from build123d import *

# Parameters (mm, degrees)
SKETCH_1_W               = 11
SKETCH_1_H               = 6.169
CUT_EXTRUDE_2_REACH      = 19.004
PATTERN_CIRCULAR_3_COUNT = 20
EXTRUDE_START            = 2
SKETCH_7_R               = 11
SKETCH_7_R_2             = 3
EXTRUDE_1_DEPTH          = 2
EXTRUDE_START_2          = -11
SKETCH_7_2_R             = 11
SKETCH_7_2_R_2           = 3
EXTRUDE_2_DEPTH          = 2
CHAMFER_1_SIZE           = 0.5


with BuildPart() as part:
    # 草图1 → 旋转1 (revolve)
    with BuildSketch(Plane.XY, mode=Mode.PRIVATE) as revolve_1_sk:
        with Locations((5.5, 6.0845)):
            Rectangle(SKETCH_1_W, SKETCH_1_H)
    revolve(revolve_1_sk.sketch.rotate(Axis((0, 0, 0), (1, 0, 0)), 90), axis=Axis((0, 0, 0), (1, 0, 0)))

    # 草图6 → 切除-拉伸2 (cut, up to next)
    with BuildSketch(Plane(origin=(0, 0, 0), x_dir=(0, 0, -1), z_dir=(1, 0, 0)), mode=Mode.PRIVATE) as cut_extrude_2_sk1:
        with BuildLine():
            Line((0.924550348, 8.86184509), (0.903216998, 8.688098898))
            ThreePointArc((0.903216998, 8.688098898), (0, 7.889), (-0.903216998, 8.688098898))
            Line((-0.903216998, 8.688098898), (-0.924550348, 8.86184509))
            ThreePointArc((-0.924550348, 8.86184509), (-1.023665877, 9.035916247), (-1.217125672, 9.087858169))
            ThreePointArc((-1.217125672, 9.087858169), (-1.345852886, 9.069688033), (-1.47430954, 9.049694601))
            Line((-1.47430954, 9.049694601), (-1.670957529, 10.651263944))
            ThreePointArc((-1.670957529, 10.651263944), (0, 10.781536192), (1.670957529, 10.651263944))
            Line((1.670957529, 10.651263944), (1.47430954, 9.049694601))
            ThreePointArc((1.47430954, 9.049694601), (1.345852886, 9.069688033), (1.217125672, 9.087858169))
            ThreePointArc((1.217125672, 9.087858169), (1.023665877, 9.035916247), (0.924550348, 8.86184509))
        make_face()
    cut_extrude_2_tool1 = extrude(cut_extrude_2_sk1.sketch, amount=CUT_EXTRUDE_2_REACH, mode=Mode.PRIVATE) & part.part
    cut_extrude_2 = cut_extrude_2_tool1.solids().sort_by_distance((0, 9.573328, 0))[0]
    add(cut_extrude_2, mode=Mode.SUBTRACT)

    # 阵列(圆周)3: 切除-拉伸2 ×20 about axis
    pattern_circular_3_axis = Axis((0, 0, 0), (1, 0, 0))
    for i in range(1, PATTERN_CIRCULAR_3_COUNT):
        add(cut_extrude_2.rotate(pattern_circular_3_axis, i * 360 / PATTERN_CIRCULAR_3_COUNT), mode=Mode.SUBTRACT)

    # 草图7 → 凸台-拉伸1 (add)
    with BuildSketch(Plane.ZY.offset(EXTRUDE_START)):
        Circle(SKETCH_7_R)
        Circle(SKETCH_7_R_2, mode=Mode.SUBTRACT)
    extrude(amount=-EXTRUDE_1_DEPTH)

    # 草图7<2> → 凸台-拉伸2 (add)
    with BuildSketch(Plane.ZY.offset(EXTRUDE_START_2)):
        Circle(SKETCH_7_2_R)
        Circle(SKETCH_7_2_R_2, mode=Mode.SUBTRACT)
    extrude(amount=-EXTRUDE_2_DEPTH)

    # 倒角1
    chamfer_1_edges = [part.edges().sort_by_distance(p)[0] for p in [
        (-2, 0, -11),
        (0, 0, -11),
        (13, 0, -11),
        (11, 0, -11),
    ]]
    chamfer(chamfer_1_edges, length=CHAMFER_1_SIZE)


solid = part.part
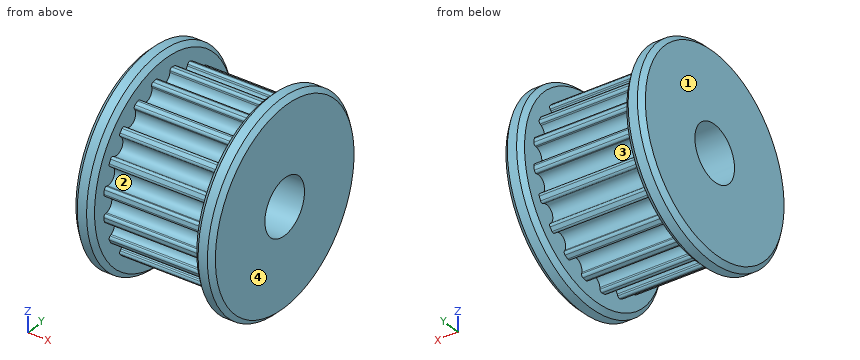
Input: part model. Units: mm. Frame: model coordinates. Face numbers are marked on the shaded views. A direction names the side the tool comes from. Give positions to 0.01 mm unless a question says otherwise; leave off trailing zeros. Write each loop counter-clockwise with the first axis right and the second up, starting at its lowest first coordinate (ties: lowest second). Pieces come first, ordered by that corner, then holes. Notation, with made-up numbers: M 55.25,81.5 L 94.25,81.5 A21 cw 94.25,104.5 Z; hole C -10.75,75.25 d7. An arc over 180 degrees is marked long. Write item = value, one per line. Start each with the question number.
1) Draft query along Z for the marked faces 1 and 2. Return one class per face: +Z half, -Z half, draft (parallel to the pull), parting line (faces both ways), or undercut.
2) Material intervals for line 1 along Y through (x, z) = (10.25, 0); line 2 along X through (y, z) = (-8.75, -3.25); line 3 along Z through (x, y) = (6, -8), sorted ascending. Write a range as [from, to].
3) First-contact query: pin 1 Ø3 at (x, z) = (8.5, -1.5) entering from +Y. Flat tip, straight axial feed; report the tip coordinate or a pass-through.
4) Reachability of the marked faces 3 and 4 from +Z, -Z, +X, -X, +Y, -Y: full face, straight path, thin tool, end or side. Return the list, or none.
5) Cut plane A-A on z = 0. Return the cut outline in (x, y).
Solved:
q1.face_1 = draft
q1.face_2 = undercut
q2.line_1 = [-7.89, -3], [3, 7.89]
q2.line_2 = [-2, 0], [11, 13]
q2.line_3 = [-4.44, -3.55], [-1.89, -0.44], [0.44, 1.89], [3.55, 4.44]
q3.pin_1 = 9.09
q4.face_3 = none
q4.face_4 = +Z, -Z, +X, +Y, -Y
q5.outline = M -2,-10.5 L -1.5,-11 L -0.5,-11 L 0,-10.5 L 0,-7.89 L 11,-7.89 L 11,-10.5 L 11.5,-11 L 12.5,-11 L 13,-10.5 L 13,-3 L -2,-3 Z; M -2,3 L 13,3 L 13,10.5 L 12.5,11 L 11.5,11 L 11,10.5 L 11,7.89 L 0,7.89 L 0,10.5 L -0.5,11 L -1.5,11 L -2,10.5 Z
